from build123d import *

# Parameters (mm, degrees)
SKETCH1_R           = 31
SKETCH1_R_2         = 29.75
BOSS_EXTRUDE1_DEPTH = 29
SKETCH2_R           = 32.5
SKETCH2_R_2         = 29.6
BOSS_EXTRUDE3_DEPTH = 35
FILLET2_R           = 2
SKETCH3_R           = 32.5
CUT_EXTRUDE1_DEPTH  = 3.5
SKETCH4_R           = 29.6
SKETCH4_R_2         = 27.5
BOSS_EXTRUDE4_DEPTH = 15
CUT_EXTRUDE2_START  = -33
SKETCH5_R           = 29.6
CUT_EXTRUDE2_DEPTH  = 33
SKETCH6_R           = 35
SKETCH6_R_2         = 29.6
BOSS_EXTRUDE5_DEPTH = 37
FILLET3_R           = 3


with BuildPart() as part:
    # Sketch1 → Boss-Extrude1 (new body)
    with BuildSketch(Plane.XY):
        with Locations(Location((0, 0, 0), (0, 0, 180))):
            Circle(SKETCH1_R)
        with Locations(Location((0, 0, 0), (0, 0, 180))):
            Circle(SKETCH1_R_2, mode=Mode.SUBTRACT)
    extrude(amount=BOSS_EXTRUDE1_DEPTH)

    # Sketch2 → Boss-Extrude3 (add)
    with BuildSketch(Plane.XY.offset(29)):
        Circle(SKETCH2_R)
        Circle(SKETCH2_R_2, mode=Mode.SUBTRACT)
    extrude(amount=-BOSS_EXTRUDE3_DEPTH)

    # Fillet2
    fillet2_edges = [part.edges().sort_by_distance(p)[0] for p in [
        (-29.6, 0, -6),
    ]]
    fillet(fillet2_edges, radius=FILLET2_R)

    # Sketch3 → Cut-Extrude1 (cut)
    with BuildSketch(Plane.XY.offset(29)):
        Circle(SKETCH3_R)
    extrude(amount=-CUT_EXTRUDE1_DEPTH, mode=Mode.SUBTRACT)

    # Sketch4 → Boss-Extrude4 (add)
    with BuildSketch(Plane.XY.offset(25.5)):
        Circle(SKETCH4_R)
        Circle(SKETCH4_R_2, mode=Mode.SUBTRACT)
    extrude(amount=-BOSS_EXTRUDE4_DEPTH)

    # Sketch5 → Cut-Extrude2 (cut)
    with BuildSketch(Plane(origin=(0, 0, 10.5), x_dir=(-1, 0, 0), z_dir=(0, 0, -1)).offset(CUT_EXTRUDE2_START)):
        with Locations(Location((0, 0, 0), (0, 0, 180))):
            Circle(SKETCH5_R)
    extrude(amount=CUT_EXTRUDE2_DEPTH, mode=Mode.SUBTRACT)

    # Sketch6 → Boss-Extrude5 (add)
    with BuildSketch(Plane.XY.offset(25.5)):
        Circle(SKETCH6_R)
        Circle(SKETCH6_R_2, mode=Mode.SUBTRACT)
    extrude(amount=-BOSS_EXTRUDE5_DEPTH)

    # Sketch7 → Revolve1 (revolve)
    with BuildSketch(Plane(origin=(0, 0, 0), x_dir=(1, 0, 0), z_dir=(0, 1, 0)), mode=Mode.PRIVATE) as revolve1_sk:
        Polygon((-27.5, 11.5), (-35, 15.830127019), (-35, 11.5), align=None)
    revolve(revolve1_sk.sketch.rotate(Axis((0, 0, -15.830127019), (0, 0, 1)), 180), axis=Axis((0, 0, -15.830127019), (0, 0, 1)))

    # Fillet3
    fillet3_edges = [part.edges().sort_by_distance(p)[0] for p in [
        (-29.6, 0, 25.5),
    ]]
    fillet(fillet3_edges, radius=FILLET3_R)


solid = part.part
CAD build for the part. Positions are in the model's coordinates, mm. A direction names the side the tool comes from. Coordinates: 2 decimals unless noted, no trailing zeros. Loops run counter-clockwise (first coordinate to the right, second up) from the corner with the lowest first, then second, coordinate; pieces in that order, holes last. Notation, with made-up numbers: (83, -7.5) - (94, -7.5) arc R22 cw to (94, 17.5) - close; hole circle Ø6 at (88.5, 11.5). An arc over 180 degrees is marked (long way). Write item = value, one per line. Start each with the question number.
Q1. Pull direction X, two halves, no side cores. Call faces 3 (the cylindrical face through (-7.587, -34.168, 5.124)), 4 (the flat face through (20, -20, -11.5)), 5 (the flat face through (-29, 16, 25.5)): pulls with the +X half, pulls with the -X half, needs draft (parallel to the pull), parting line crosses it, or undercut.
Q2. Which spindle directions (+Z, -Z, +X, -X, +Y, -Y) get a long thin tool onto all of the face, cutting with end or side? Do faces 1 (the cylindrical face through (-6.4, -28.9, 5.7)), 2 (the conical face through (-6.06, -27.3, -11.77)). Say none if no direction does.
Q3. Flat gauge pins, fed straight in: pin 1 Ø12 at (y, z) = (-20.5, 15) entering from +X; pin 2 Ø3 at (y, z) = (-27.5, 20) entering from -X; pin 3 Ø6 at (x, z) = (21.5, 11.5) entering from +Y; pin 4 Ø18 at (x, y) = (10, 3.5) entering from +Z. Where does each tip first touch, or does it go through?
Q4. Cut at A-A, the plane x = 0. List the corners of the cut face in (y, z).
Q5. Cut at C-C, the plane z = 5.5. List the corners of the cut face in (x, y), then the cut area to 3 significant figures.
Q6. Drill centre lines: L1, parallel to X at y = 1, z = 16; L2, parallel to Y at x = 0, z = 0; L3, parallel to Y at x = 20, z = 7. Where is each one in solid material? Low to high.
Computed:
q1.face_3 = parting line crosses it
q1.face_4 = undercut
q1.face_5 = needs draft
q2.face_1 = +Z
q2.face_2 = -Z
q3.pin_1 = 31.86
q3.pin_2 = -23.43
q3.pin_3 = 29.71
q3.pin_4 = through
q4.outline = (-35, -15.83) - (-27.5, -11.5) - (-29.6, -11.5) - (-29.6, 22.5) arc R3 ccw to (-32.6, 25.5) - (-35, 25.5) - close; (27.5, -11.5) - (35, -15.83) - (35, 25.5) - (32.6, 25.5) arc R3 ccw to (29.6, 22.5) - (29.6, -11.5) - close
q5.outline = circle Ø70 at (0, 0); hole circle Ø59.2 at (0, 0)
q5.area = 1,100 mm²
q6.L1 = -34.99 to -29.58, 29.58 to 34.99
q6.L2 = -35 to -29.6, 29.6 to 35
q6.L3 = -28.72 to -21.82, 21.82 to 28.72
